Geometry check sheet. Reference: drawing and pictorial views, mm from the part's lowest x, y, z. A direction names the side the tool comes from. Give positions to 0.01 mm unless a question says otherwise; leave off trailing zeros. Order: outer loops, then holes, each group sorted by start corner. A loop starts at its lowest first (then second) coordinate and runs counter-clockwise, first axis right, second up.
Item 1: Sectioned sample at B-B on y = 11.5. Record the boundary of the cut face in (x, z), and give its area (3 significant figures).
Item 2: Sectioned sample at C-C on z = 7. Record the boundary of the cut face in (x, y), and give its area (3 significant figures).
Item 3: Access from +Z, -Z, +X, -X, +Y, -Y to the whole of each face (thin tool, end or side, straight path). Record for the marked faces 1, 2, 3 and 4.
Item 4: Material ranges on line 1 along Z through (x, y) = (10, 13.75); line 2 along X through (y, z) = (7.5, 10.5), recorded low to high.
Item 5: Sectioned sample at D-D on z = 4. Record the boundary of the cut face in (x, y).
Item 6: Sectioned sample at A-A on x = 7.5. Record the boundary of the cut face in (y, z), and give its area (3 significant figures).
Item 7: Gauge pin test, flat ends, axial feed: P1, Ø2, axis at y = 12, z = 17, coming from the -X side; P2, Ø1.5, axis at x = 2, z = 12, coming from the -Y side; P3, Ø5, axis at x = 13, z = 20.5, coming from the +Y side. Record the tip position at first contact, or that the pin passes through.
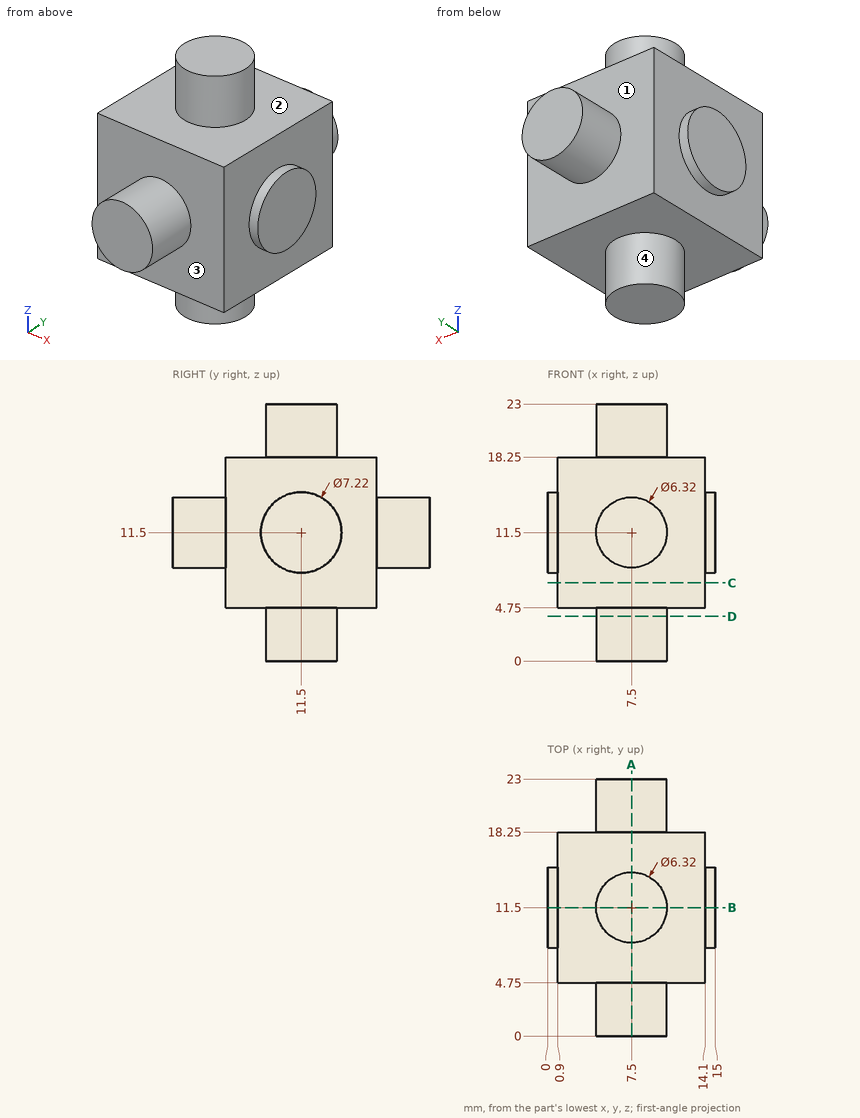
Report:
1. outline: (0, 7.89) - (0.9, 7.89) - (0.9, 4.75) - (4.34, 4.75) - (4.34, 0) - (10.66, 0) - (10.66, 4.75) - (14.1, 4.75) - (14.1, 7.89) - (15, 7.89) - (15, 15.11) - (14.1, 15.11) - (14.1, 18.25) - (10.66, 18.25) - (10.66, 23) - (4.34, 23) - (4.34, 18.25) - (0.9, 18.25) - (0.9, 15.11) - (0, 15.11) - close
1. area: 251 mm2
2. outline: (0.9, 4.75) - (14.1, 4.75) - (14.1, 18.25) - (0.9, 18.25) - close
2. area: 178 mm2
3. face 1: +Y
3. face 2: +Z
3. face 3: -Y
3. face 4: -Z
4. line 1: z = 4.75 to 18.25
4. line 2: x = 0.9 to 14.1
5. outline: circle Ø6.32 at (7.5, 11.5)
6. outline: (0, 8.34) - (4.75, 8.34) - (4.75, 4.75) - (8.34, 4.75) - (8.34, 0) - (14.66, 0) - (14.66, 4.75) - (18.25, 4.75) - (18.25, 8.34) - (23, 8.34) - (23, 14.66) - (18.25, 14.66) - (18.25, 18.25) - (14.66, 18.25) - (14.66, 23) - (8.34, 23) - (8.34, 18.25) - (4.75, 18.25) - (4.75, 14.66) - (0, 14.66) - close
6. area: 302 mm2
7. P1: stops at x = 0.9
7. P2: stops at y = 4.75
7. P3: stops at y = 18.25
